Work out the finished part from the listing and answer in its coordinate system (mm). A direction names the side the tool comes from. Round coordinates to 2 decimals unless told otherwise and drop trailing zeros. Order: outer loops, then holes, each group sorted by start corner. A loop starts at its lowest first (then second) coordinate and runs counter-clockwise, first axis right, second up. Notation, with made-up numbers: (-20.5, 40.5) - (9.5, 40.5) arc R19 ccw to (9.5, 48.5) - close; hole circle Ø4 at (57.25, -2). An arc over 180 degrees is marked (long way). Put each result on its own line as item: value.
```python
from build123d import *

# Parameters (mm, degrees)
SKETCH_1_W                = 26
SKETCH_1_H                = 9
EXTRUDE_1_DEPTH           = 10
SKETCH_2_R                = 3.6
CUT_EXTRUDE_1_DEPTH       = 18.007351352
EXTRUDE_2_DEPTH           = 26
CUT_EXTRUDE_2_DEPTH       = 7
SKETCH_7_W                = 8.5
SKETCH_7_H                = 9
EXTRUDE_3_DEPTH           = 40
SKETCH_8_R                = 1.75
CUT_EXTRUDE_3_DEPTH       = 40
SKETCH_9_W                = 3.5
SKETCH_9_H                = 34
CUT_EXTRUDE_4_DEPTH       = 7
CUT_EXTRUDE_12_DEPTH      = 50.979995998
PATTERN_START             = -4.5
PATTERN_LINEAR_2_DEPTH    = 9
SKETCH_22_W               = 8.5
SKETCH_22_H               = 34
CUT_EXTRUDE_13_DEPTH      = 4
CUT_EXTRUDE_17_DEPTH      = 58.168610268
CUT_EXTRUDE_17_DEPTH_BACK = 58.168610268
SKETCH_27_W               = 4
SKETCH_27_H               = 28.3452151
CUT_EXTRUDE_18_DEPTH      = 52.168838173
CUT_EXTRUDE_18_DEPTH_BACK = 12
F_2_0MM_1_D               = 1.5
F_2_0MM_1_DEPTH           = 5
F_2_0MM_1_TIP             = 0.450645464
F_2_0MM_2_D               = 1.5
F_2_0MM_2_DEPTH           = 4
F_2_0MM_2_TIP             = 0.450645464


# Read off the part's stored shape, not the designer's step: 阵列(线性)2
with BuildPart() as part:
    # 草图1 → 凸台-拉伸1 (new body)
    with BuildSketch(Plane.XY):
        Rectangle(SKETCH_1_W, SKETCH_1_H)
    extrude(amount=-EXTRUDE_1_DEPTH)

    # 草图2 → 切除-拉伸1 (cut, through all)
    with BuildSketch(Plane.XY):
        with Locations((8.5, 0)):
            Circle(SKETCH_2_R)
        with Locations(Location((-8.5, 0, 0), (0, 0, 180))):
            Circle(SKETCH_2_R)
    extrude(amount=-CUT_EXTRUDE_1_DEPTH, mode=Mode.SUBTRACT)

    # 草图5 → 凸台-拉伸2 (add, through all)
    with BuildSketch(Plane.ZY.offset(13)):
        with BuildLine():
            Line((0, 4.5), (-10, 4.5))
            Line((-10, 4.5), (-10, 8.301419967))
            Line((-10, 8.301419967), (-10, 30.5))
            ThreePointArc((-10, 30.5), (-9.707106781, 31.207106781), (-9, 31.5))
            Line((-9, 31.5), (-8, 31.5))
            Line((-8, 31.5), (-8, 20.1))
            ThreePointArc((-8, 20.1), (-7.53137085, 18.96862915), (-6.4, 18.5))
            Line((-6.4, 18.5), (-2.5, 18.5))
            ThreePointArc((-2.5, 18.5), (-0.732233047, 17.767766953), (0, 16))
            Line((0, 16), (0, 4.5))
        make_face()
    extrude(amount=-EXTRUDE_2_DEPTH)

    # 草图5<2> → 切除-拉伸2 (cut)
    with BuildSketch(Plane.ZY.offset(13)):
        with BuildLine():
            Line((0, 4.5), (-10, 4.5))
            Line((-10, 4.5), (-10, 8.301419967))
            Line((-10, 8.301419967), (-10, 30.5))
            ThreePointArc((-10, 30.5), (-9.707106781, 31.207106781), (-9, 31.5))
            Line((-9, 31.5), (-8, 31.5))
            Line((-8, 31.5), (-8, 20.1))
            ThreePointArc((-8, 20.1), (-7.53137085, 18.96862915), (-6.4, 18.5))
            Line((-6.4, 18.5), (-2.5, 18.5))
            ThreePointArc((-2.5, 18.5), (-0.732233047, 17.767766953), (0, 16))
            Line((0, 16), (0, 4.5))
        make_face()
    cut_extrude_2 = extrude(amount=-CUT_EXTRUDE_2_DEPTH, mode=Mode.SUBTRACT)

    # 镜向1: 切除-拉伸2 across plane
    add(cut_extrude_2.mirror(Plane(origin=(0, 0, 0), x_dir=(0, 0, 1), z_dir=(1, 0, 0))), mode=Mode.SUBTRACT)

    # 草图7 → 凸台-拉伸3 (add)
    with BuildSketch(Plane.XY):
        with Locations((8.75, 0)):
            Rectangle(SKETCH_7_W, SKETCH_7_H)
    extrude(amount=EXTRUDE_3_DEPTH)

    # 草图8 → 切除-拉伸3 (cut)
    with BuildSketch(Plane.XY.offset(40)):
        with Locations((8.5, 0)):
            Circle(SKETCH_8_R)
    extrude(amount=-CUT_EXTRUDE_3_DEPTH, mode=Mode.SUBTRACT)

    # 草图9 → 切除-拉伸4 (cut)
    with BuildSketch(Plane(origin=(0, 4.5, 0), x_dir=(1, 0, 0), z_dir=(0, 1, 0))):
        with Locations((8.75, -20)):
            Rectangle(SKETCH_9_W, SKETCH_9_H)
    extrude(amount=-CUT_EXTRUDE_4_DEPTH, mode=Mode.SUBTRACT)

    # 草图10 → 切除-拉伸12 (cut, through all)
    with BuildSketch(Plane(origin=(0, 4.5, 0), x_dir=(1, 0, 0), z_dir=(0, 1, 0))):
        Polygon((5.625, -40), (5.625, -40.330435371), (4.5, -40.739901884), (4.5, -39.590533486), align=None)
    extrude(amount=-CUT_EXTRUDE_12_DEPTH, mode=Mode.SUBTRACT)

    # 阵列(线性)2 outline → 阵列(线性)2 (cut)
    with BuildSketch(Plane(origin=(0, 0, 0), x_dir=(1, 0, 0), z_dir=(0, 1, 0)).offset(PATTERN_START)):
        Polygon((5.625, -10.485305161), (5.625, -10.154869791), (4.5, -9.745403277), (4.5, -10.894771675), align=None)
        Polygon((5.625, -38.429203673), (4.5, -38.01973716), (4.5, -39.169105557), (5.625, -38.759639044), align=None)
        Polygon((5.625, -36.858407346), (4.5, -36.448940833), (4.5, -37.598309231), (5.625, -37.188842717), align=None)
        Polygon((5.625, -35.28761102), (4.5, -34.878144506), (4.5, -36.027512904), (5.625, -35.61804639), align=None)
        Polygon((5.625, -33.716814693), (4.5, -33.307348179), (4.5, -34.456716577), (5.625, -34.047250063), align=None)
        Polygon((5.625, -32.146018366), (4.5, -31.736551852), (4.5, -32.88592025), (5.625, -32.476453737), align=None)
        Polygon((5.625, -30.575222039), (4.5, -30.165755526), (4.5, -31.315123923), (5.625, -30.90565741), align=None)
        Polygon((5.625, -29.004425712), (4.5, -28.594959199), (4.5, -29.744327597), (5.625, -29.334861083), align=None)
        Polygon((5.625, -27.433629386), (4.5, -27.024162872), (4.5, -28.17353127), (5.625, -27.764064756), align=None)
        Polygon((5.625, -25.862833059), (4.5, -25.453366545), (4.5, -26.602734943), (5.625, -26.193268429), align=None)
        Polygon((5.625, -24.292036732), (4.5, -23.882570219), (4.5, -25.031938616), (5.625, -24.622472103), align=None)
        Polygon((5.625, -22.721240405), (4.5, -22.311773892), (4.5, -23.461142289), (5.625, -23.051675776), align=None)
        Polygon((5.625, -21.150444078), (4.5, -20.740977565), (4.5, -21.890345963), (5.625, -21.480879449), align=None)
        Polygon((5.625, -19.579647752), (4.5, -19.170181238), (4.5, -20.319549636), (5.625, -19.910083122), align=None)
        Polygon((5.625, -18.008851425), (4.5, -17.599384911), (4.5, -18.748753309), (5.625, -18.339286795), align=None)
        Polygon((5.625, -16.438055098), (4.5, -16.028588585), (4.5, -17.177956982), (5.625, -16.768490469), align=None)
        Polygon((5.625, -14.867258771), (4.5, -14.457792258), (4.5, -15.607160655), (5.625, -15.197694142), align=None)
        Polygon((5.625, -13.296462444), (4.5, -12.886995931), (4.5, -14.036364329), (5.625, -13.626897815), align=None)
        Polygon((5.625, -11.725666118), (4.5, -11.316199604), (4.5, -12.465568002), (5.625, -12.056101488), align=None)
    extrude(amount=PATTERN_LINEAR_2_DEPTH, mode=Mode.SUBTRACT)

    # 草图22 → 切除-拉伸13 (cut)
    with BuildSketch(Plane(origin=(0, 4.5, 0), x_dir=(1, 0, 0), z_dir=(0, 1, 0))):
        with Locations((8.75, -20)):
            Rectangle(SKETCH_22_W, SKETCH_22_H)
    extrude(amount=-CUT_EXTRUDE_13_DEPTH, mode=Mode.SUBTRACT)

    # 草图27 → 切除-拉伸17 (cut, two sides: drawn at the far end of the back side and taken through both)
    with BuildSketch(Plane.ZY.offset(13).offset(-CUT_EXTRUDE_17_DEPTH_BACK)):
        with Locations((-8, 18.67260755)):
            Rectangle(SKETCH_27_W, SKETCH_27_H)
    extrude(amount=CUT_EXTRUDE_17_DEPTH + CUT_EXTRUDE_17_DEPTH_BACK, mode=Mode.SUBTRACT)

    # 草图5<5> → 切除-拉伸18 (cut, two sides: drawn at the far end of the back side and taken through both)
    with BuildSketch(Plane.ZY.offset(13).offset(-CUT_EXTRUDE_18_DEPTH_BACK)):
        with BuildLine():
            Line((0, 4.5), (-10, 4.5))
            Line((-10, 4.5), (-10, 8.301419967))
            Line((-10, 8.301419967), (-10, 30.5))
            ThreePointArc((-10, 30.5), (-9.707106781, 31.207106781), (-9, 31.5))
            Line((-9, 31.5), (-8, 31.5))
            Line((-8, 31.5), (-8, 20.1))
            ThreePointArc((-8, 20.1), (-7.53137085, 18.96862915), (-6.4, 18.5))
            Line((-6.4, 18.5), (-2.5, 18.5))
            ThreePointArc((-2.5, 18.5), (-0.732233047, 17.767766953), (0, 16))
            Line((0, 16), (0, 4.5))
        make_face()
    extrude(amount=CUT_EXTRUDE_18_DEPTH + CUT_EXTRUDE_18_DEPTH_BACK, mode=Mode.SUBTRACT)

    # Ø2.0mm 暗销孔1
    with Locations(Plane(origin=(0, 0, -6), x_dir=(-1, 0, 0), z_dir=(0, 0, -1))):
        with Locations((-2.5, 13.5), (-2.5, 8.5)):
            Hole(F_2_0MM_1_D / 2, depth=F_2_0MM_1_DEPTH)
            with Locations((0, 0, -(F_2_0MM_1_DEPTH + F_2_0MM_1_TIP / 2))):  # 118° drill point
                Cone(0, F_2_0MM_1_D / 2, F_2_0MM_1_TIP, mode=Mode.SUBTRACT)

    # Ø2.0mm 暗销孔2
    with Locations(Plane.ZY.offset(1)):
        with Locations((-3, 11)):
            Hole(F_2_0MM_2_D / 2, depth=F_2_0MM_2_DEPTH)
            with Locations((0, 0, -(F_2_0MM_2_DEPTH + F_2_0MM_2_TIP / 2))):  # 118° drill point
                Cone(0, F_2_0MM_2_D / 2, F_2_0MM_2_TIP, mode=Mode.SUBTRACT)


solid = part.part
```
1) Straight lines are drawn through the part: L1, parallel to X at y = 8.5, z = -2.4; L2, parallel to Z at x = 8.5, y = 4; L3, parallel to Y at x = 2.5, z = -3.4. For each, find the intervals that lie inside material, in ascending order. Write a range as from..to.
Findings below:
L1: x = -1..1.75, 3.25..6
L2: z = -10..3, 37..40
L3: y = -4.5..7.75, 9.25..10.37, 11.63..12.75, 14.25..18.5
2) A cutting plane is placed at D-D on x = 9.75. Write down the section's boundary in (y, z).
Findings below:
outline: (-4.5, -10) - (-3.38, -10) - (-3.38, 0) - (-1.22, 0) - (-1.22, 3) - (-2.5, 3) - (-2.5, 37) - (-1.22, 37) - (-1.22, 40) - (-4.5, 40) - close; (1.22, 0) - (3.38, 0) - (3.38, -10) - (4.5, -10) - (4.5, 3) - (1.22, 3) - close; (1.22, 37) - (4.5, 37) - (4.5, 40) - (1.22, 40) - close
3) A cutting plane is placed at B-B on z = 6.5. Write down the section's boundary in (x, y), then the cut area to 3 significant figures.
Findings below:
outline: (4.5, -4.5) - (13, -4.5) - (13, 0.5) - (10.5, 0.5) - (10.5, -2.5) - (7, -2.5) - (7, -0.9) arc R1.75 cw to (6.82, 0.5) - (4.5, 0.5) - close
area: 31.7 mm2
4) A cutting plane is placed at C-C on y = 0. Give the number of separate pieces and of enclosed holes in the cut face, then the cut area to 3 significant figures.
Findings below:
separate pieces: 3
enclosed holes: 0
area: 291 mm2
5) For a pull along Z with two mould halves and no side action, classify faces 6 (the conical face through (2.43, 8.61, -0.63)), 7 (the flat face through (5.07, -2.035, 9.953)), 8 (the flat face through (6, 12, -3)) as pulls with the +Z half, pulls with the -Z half, needs draft (parallel to the pull), parting line crosses it, or undercut.
Findings below:
face 6: pulls with the -Z half
face 7: undercut
face 8: needs draft
6) A cutting plane is placed at A-A on x = -8.5. Write down the section's boundary in (y, z).
Findings below:
outline: (-4.5, -10) - (-3.6, -10) - (-3.6, 0) - (-4.5, 0) - close; (3.6, -10) - (4.5, -10) - (4.5, 0) - (3.6, 0) - close
7) Given pin 1 Ø2 at (x, y) = (10, -0.5) entering from -Z; pin 2 Ø1.5 at (x, y) = (4.5, 5) entering from +Z; pin 3 Ø5.5 at (x, y) = (-2, 8.5) entering from +Z, each flat-ended and moving along its own axis, determine where each tip first touches the part or whether it passes through.
Findings below:
pin 1: stops at z = 0
pin 2: stops at z = 39.79
pin 3: stops at z = 0
8) For faces 1 (the cylindrical face through (2, 18, -1)), 2 (the cylindrical face through (2.402, 9.244, -3.465)), 3 (the flat face through (4.5, -1, 4)), 4 (the flat face through (5.07, -2.035, 14.665)), 5 (the flat face through (9, -2.5, 20)), determine the directions among +Z, -Z, +X, -X, +Y, -Y from which every point of the face is accessible in a straight line to the end or side of a thin tool.
Findings below:
face 1: +Z, +X, -X, +Y
face 2: -Z
face 3: +Z, -X, +Y, -Y
face 4: -X, +Y, -Y
face 5: +Y
